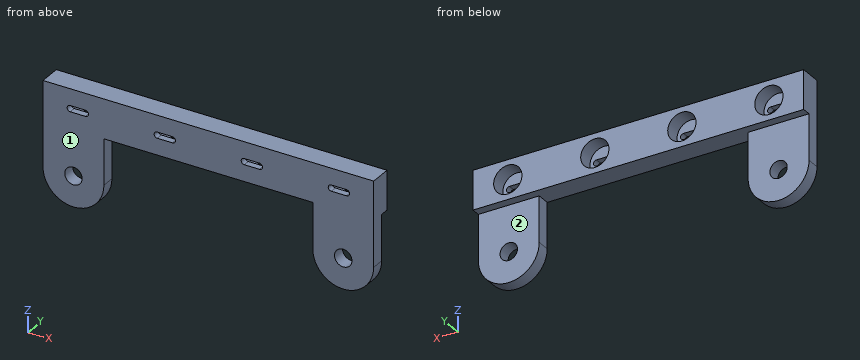
```python
from build123d import *

# Parameters (mm, degrees)
SKETCH1_R           = 2
BOSS_EXTRUDE1_DEPTH = 3
SKETCH2_W           = 76
SKETCH2_H           = 9
BOSS_EXTRUDE2_DEPTH = 2
SKETCH3_R           = 3.25
CUT_EXTRUDE1_DEPTH  = 3.5
CUT_EXTRUDE2_REACH  = 82.564


with BuildPart() as part:
    # Sketch1 → Boss-Extrude1 (new body)
    with BuildSketch(Plane(origin=(0, 0, 0), x_dir=(1, 0, 0), z_dir=(0, 1, 0))):
        with BuildLine():
            ThreePointArc((76, 19.5), (69, 26.5), (62, 19.5))
            Line((62, 19.5), (62, 9))
            Line((62, 9), (14, 9))
            Line((14, 9), (14, 19.5))
            ThreePointArc((14, 19.5), (7, 26.5), (0, 19.5))
            Line((0, 19.5), (0, 0))
            Line((0, 0), (76, 0))
            Line((76, 0), (76, 19.5))
        make_face()
        with Locations(Location((69, 19.5, 0), (0, 0, 270))):
            Circle(SKETCH1_R, mode=Mode.SUBTRACT)
        with Locations(Location((7, 19.5, 0), (0, 0, 270))):
            Circle(SKETCH1_R, mode=Mode.SUBTRACT)
    extrude(amount=BOSS_EXTRUDE1_DEPTH)

    # Sketch2 → Boss-Extrude2 (add)
    with BuildSketch(Plane(origin=(0, 3, 0), x_dir=(1, 0, 0), z_dir=(0, 1, 0))):
        with Locations((38, 4.5)):
            Rectangle(SKETCH2_W, SKETCH2_H)
    extrude(amount=BOSS_EXTRUDE2_DEPTH)

    # Sketch3 → Cut-Extrude1 (cut)
    with BuildSketch(Plane(origin=(0, 5, 0), x_dir=(1, 0, 0), z_dir=(0, 1, 0))):
        with Locations(Location((8, 4.5, 0), (0, 0, 270))):
            Circle(SKETCH3_R)
        with Locations(Location((28, 4.5, 0), (0, 0, 270))):
            Circle(SKETCH3_R)
        with Locations(Location((48, 4.5, 0), (0, 0, 270))):
            Circle(SKETCH3_R)
        with Locations(Location((68, 4.5, 0), (0, 0, 270))):
            Circle(SKETCH3_R)
    extrude(amount=-CUT_EXTRUDE1_DEPTH, mode=Mode.SUBTRACT)

    # Sketch4 → Cut-Extrude2 (cut, up to next)
    with BuildSketch(Plane(origin=(0, 1.5, 0), x_dir=(1, 0, 0), z_dir=(0, 1, 0)), mode=Mode.PRIVATE) as cut_extrude2_sk1:
        with BuildLine():
            Line((6.25, 5.2), (9.75, 5.2))
            ThreePointArc((9.75, 5.2), (10.45, 4.5), (9.75, 3.8))
            Line((9.75, 3.8), (6.25, 3.8))
            ThreePointArc((6.25, 3.8), (5.55, 4.5), (6.25, 5.2))
        make_face()
    cut_extrude2_tool1 = extrude(cut_extrude2_sk1.sketch, amount=-CUT_EXTRUDE2_REACH, mode=Mode.PRIVATE) & part.part
    # Sketch4 → Cut-Extrude2 (cut, up to next)
    with BuildSketch(Plane(origin=(0, 1.5, 0), x_dir=(1, 0, 0), z_dir=(0, 1, 0)), mode=Mode.PRIVATE) as cut_extrude2_sk2:
        with BuildLine():
            Line((26.25, 5.2), (29.75, 5.2))
            ThreePointArc((29.75, 5.2), (30.45, 4.5), (29.75, 3.8))
            Line((29.75, 3.8), (26.25, 3.8))
            ThreePointArc((26.25, 3.8), (25.55, 4.5), (26.25, 5.2))
        make_face()
    cut_extrude2_tool2 = extrude(cut_extrude2_sk2.sketch, amount=-CUT_EXTRUDE2_REACH, mode=Mode.PRIVATE) & part.part
    # Sketch4 → Cut-Extrude2 (cut, up to next)
    with BuildSketch(Plane(origin=(0, 1.5, 0), x_dir=(1, 0, 0), z_dir=(0, 1, 0)), mode=Mode.PRIVATE) as cut_extrude2_sk3:
        with BuildLine():
            Line((46.25, 5.2), (49.75, 5.2))
            ThreePointArc((49.75, 5.2), (50.45, 4.5), (49.75, 3.8))
            Line((49.75, 3.8), (46.25, 3.8))
            ThreePointArc((46.25, 3.8), (45.55, 4.5), (46.25, 5.2))
        make_face()
    cut_extrude2_tool3 = extrude(cut_extrude2_sk3.sketch, amount=-CUT_EXTRUDE2_REACH, mode=Mode.PRIVATE) & part.part
    # Sketch4 → Cut-Extrude2 (cut, up to next)
    with BuildSketch(Plane(origin=(0, 1.5, 0), x_dir=(1, 0, 0), z_dir=(0, 1, 0)), mode=Mode.PRIVATE) as cut_extrude2_sk4:
        with BuildLine():
            Line((66.25, 5.2), (69.75, 5.2))
            ThreePointArc((69.75, 5.2), (70.45, 4.5), (69.75, 3.8))
            Line((69.75, 3.8), (66.25, 3.8))
            ThreePointArc((66.25, 3.8), (65.55, 4.5), (66.25, 5.2))
        make_face()
    cut_extrude2_tool4 = extrude(cut_extrude2_sk4.sketch, amount=-CUT_EXTRUDE2_REACH, mode=Mode.PRIVATE) & part.part
    add(cut_extrude2_tool1.solids().sort_by_distance((8, 1.5, -4.5))[0], mode=Mode.SUBTRACT)
    add(cut_extrude2_tool2.solids().sort_by_distance((28, 1.5, -4.5))[0], mode=Mode.SUBTRACT)
    add(cut_extrude2_tool3.solids().sort_by_distance((48, 1.5, -4.5))[0], mode=Mode.SUBTRACT)
    add(cut_extrude2_tool4.solids().sort_by_distance((68, 1.5, -4.5))[0], mode=Mode.SUBTRACT)


solid = part.part
```
Verification items for the finished model (mm, model axes). Face numbers are marked on the shaded views. A direction names the side the tool comes from. Round coordinates to 2 decimals unless told otherwise and drop trailing zeros. Order: outer loops, then holes, each group sorted by start corner. A loop starts at its lowest first (then second) coordinate and runs counter-clockwise, first axis right, second up. Notation, with made-up numbers: (74, -2) -> (82, -2) arc R8 cw to (82, 3) -> close; hole circle Ø1 at (-8.5, -32.5). An arc over 180 degrees is marked (long way). Put each result on its own line as item: value. Start each with the question number.
(1) Material ranges on line 1 along X through (y, z) = (2.45, -4.5); line 2 along X through (y, z) = (2, -19.5); line 3 along Y through (x, z) = (12, -9.25), recorded low to high.
(2) Depth check by flat-ended pin: pin 1 Ø1.6 at (x, y) = (8, 1) entering from -Z; pin 2 Ø1.5 at (x, y) = (43, 2.5) entering from -Z; pin 3 Ø4 at (x, z) = (5, -19) entering from +Y. Enter the tip coordinate at first touch or a pass-through.
(3) Section check A-A (z = -15.5). Enter the section's corners in (x, y), then the cut area to 3 significant figures.
(4) Section check D-D (x = 69). Enter the section's corners in (y, z), then the cut area to 3 significant figures.
(5) Section check C-C (y = 3.65). Enter the section's corners in (x, z).
(6) Section check B-B (x = 48). Enter the section's corners in (y, z), then the cut area to 4 significant figures.
(7) Tool access check on the marked faces 1 and 2. Record the directions out of +Z, -Z, +X, -X, +Y, -Y that give a thin tool (end or side, any length) a straight path to the whole face; none if there is none.
Completed:
1. line 1: x = 0 to 4.75, 11.25 to 24.75, 31.25 to 44.75, 51.25 to 64.75, 71.25 to 76
1. line 2: x = 0 to 5, 9 to 14, 62 to 67, 71 to 76
1. line 3: y = 0 to 3
2. pin 1: stops at z = -26.5
2. pin 2: stops at z = -9
2. pin 3: stops at y = 3
3. outline: (0, 0) -> (14, 0) -> (14, 3) -> (0, 3) -> close; (62, 0) -> (76, 0) -> (76, 3) -> (62, 3) -> close
3. area: 84.0 mm2
4. outline: (0, -26.5) -> (3, -26.5) -> (3, -21.5) -> (0, -21.5) -> close; (0, -17.5) -> (3, -17.5) -> (3, -9) -> (5, -9) -> (5, -7.59) -> (1.5, -7.59) -> (1.5, -5.2) -> (0, -5.2) -> close; (0, -3.8) -> (1.5, -3.8) -> (1.5, -1.41) -> (5, -1.41) -> (5, 0) -> (0, 0) -> close
4. area: 61.8 mm2
5. outline: (0, -9) -> (76, -9) -> (76, 0) -> (0, 0) -> close; hole circle Ø6.5 at (8, -4.5); hole circle Ø6.5 at (28, -4.5); hole circle Ø6.5 at (48, -4.5); hole circle Ø6.5 at (68, -4.5)
6. outline: (0, -9) -> (5, -9) -> (5, -7.75) -> (1.5, -7.75) -> (1.5, -5.2) -> (0, -5.2) -> close; (0, -3.8) -> (1.5, -3.8) -> (1.5, -1.25) -> (5, -1.25) -> (5, 0) -> (0, 0) -> close
6. area: 20.15 mm2
7. face 1: +Z, -Z, +X, -X, -Y
7. face 2: -Z, +X, -X, +Y
